Could you check a few things on this drawing? It's one solid part, dimensions in mm from its lowest x, y, z. A direction names the side the tool comes from. Round coordinates to 2 decimals unless told otherwise and drop trailing zeros. Loops run counter-clockwise (first coordinate to the right, second up) from the corner with the lowest first, then second, coordinate; pieces in that order, holes last. Notation, with made-up numbers: M 9,86.5 L 18,86.5 A25 cw 18,98.5 Z; hole C -1.75,22.25 d8. An arc over 180 degrees is marked long. Answer as a JSON object with one key per item and string values.
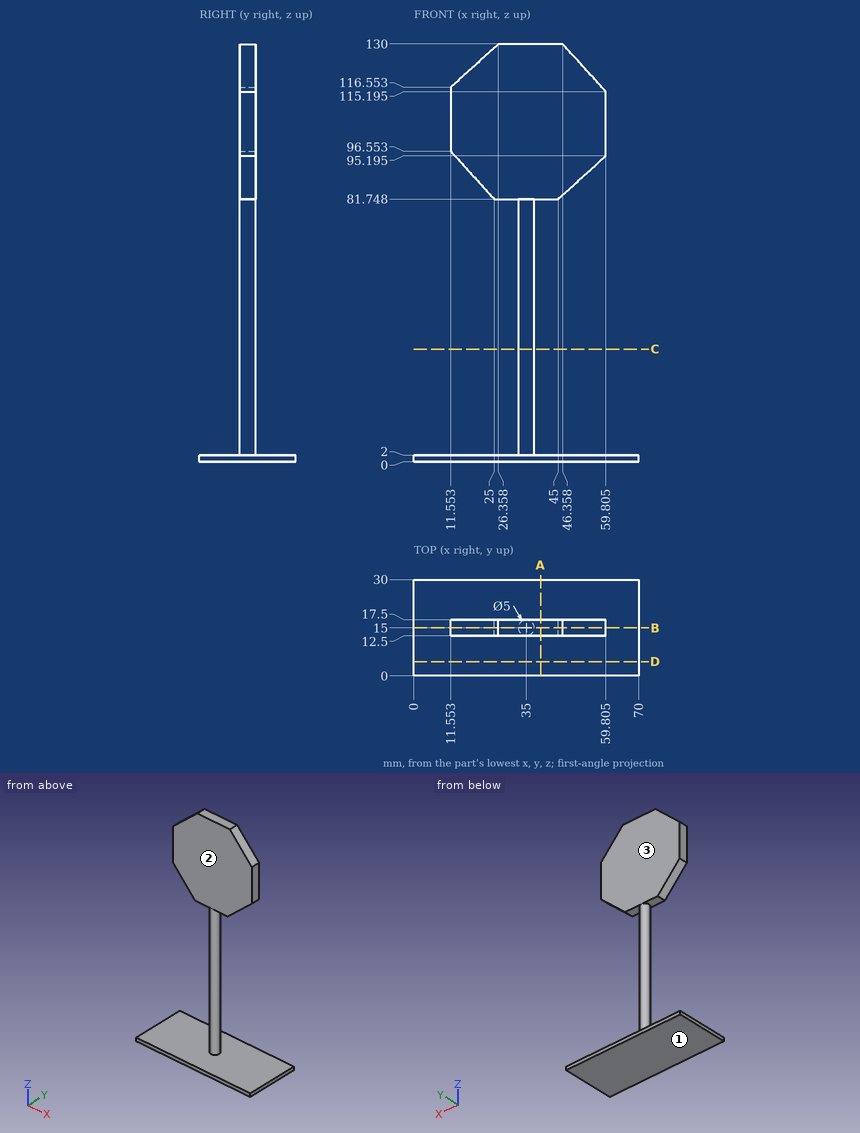
Item 1: I want a section at A-A, the plane x = 39.5. Please give me the cut outline in (y, z), then the cut area to 3 significant figures.
Resolved:
{"outline": "M 0,0 L 30,0 L 30,2 L 0,2 Z; M 12.5,81.75 L 17.5,81.75 L 17.5,130 L 12.5,130 Z", "area": "301 mm²"}
Item 2: I'm going to push flat-ended pins straight in: pin 1 Ø8 at (y, z) = (14, 76) entering from +X; pin 2 Ø10 at (x, z) = (37.5, 95.5) entering from -Y; pin 3 Ø10 at (x, z) = (28, 56) entering from -Y. Where does each tip first touch, or does it pass through?
Resolved:
{"pin 1": "x = 37.5", "pin 2": "y = 12.5", "pin 3": "y = 13.5"}
Item 3: Please list where these lines run through material, in increasing order: probe 1 along Z at (x, y) = (30, 12.75); probe 2 along Z at (x, y) = (42, 11); probe 3 along Y at (x, z) = (21.5, 93). Write a range as from..to.
Resolved:
{"probe 1": "0..2, 81.75..130", "probe 2": "0..2", "probe 3": "12.5..17.5"}
Item 4: I want a section at D-D, the plane y = 4.5. Please give me the cut outline in (x, z), then the cut area to 3 significant figures.
Resolved:
{"outline": "M 0,0 L 70,0 L 70,2 L 0,2 Z", "area": "140 mm²"}
Item 5: I want a section at C-C, the plane z = 35. Please give me the cut outline in (x, y), then the cut area to 3 significant figures.
Resolved:
{"outline": "C 35,15 d5", "area": "19.6 mm²"}
Item 6: I want a section at B-B, the plane y = 15. Please give me the cut outline in (x, z) (1 decimal).
Resolved:
{"outline": "M 0,0 L 70,0 L 70,2 L 37.5,2 L 37.5,81.7 L 45,81.7 L 59.8,95.2 L 59.8,115.2 L 46.4,130 L 26.4,130 L 11.6,116.6 L 11.6,96.6 L 25,81.7 L 32.5,81.7 L 32.5,2 L 0,2 Z"}
Item 7: On a 3-axis mill with a long thin cutter (end or side, diameter ignored), from which of +Z, -Z, +X, -X, +Y, -Y can I reach the whole of each face in a straight line? I mean the marked faces 1, 2 and 3. Say none if no direction works.
Resolved:
{"face 1": "-Z, +X, -X, +Y, -Y", "face 2": "+Z, +X, -X, -Y", "face 3": "+Z, +X, -X, +Y"}
